Work out the finished part from the listing and answer in its coordinate system (mm). A direction names the side the tool comes from. Coordinates: 2 decimals unless noted, no trailing zeros. Order: outer loops, then holes, each group sorted by start corner. A loop starts at its lowest first (then second) coordinate and runs counter-clockwise, first axis right, second up. Notation, with made-up numbers: M 9.5,52 L 59.5,52 A32 ccw 59.5,83 Z; hole C 5,39 d7. An arc over 180 degrees is marked long. Write item = value, one per line. Start each with the question number.
Q1. Find section C-C on y = 1.2. Give the vertices of the cut face in (x, z).
Q2. Find section B-B on x = 3.75. Give the vertices of the cut face in (y, z), and give its area (4 significant figures).
Q3. A tool of negligible diameter and unlimited length cuts with its end or side. For faces 4 (the flat face through (7.5, 1, -51)), 5 (the cylindrical face through (3.8, 1.2, -97.5)), from which of +Z, -Z, +X, -X, +Y, -Y can it reach the whole face along a straight path? Write none if from no direction.
Q4. Determine the mould class of faces 1 (the cylindrical face through (3.67, 1.23, -103.75)), 2 (the flat face through (1.25, 1, -51)), 3 (the flat face through (0, 1, -49)) for opening direction Z: released by +Z, released by -Z, zero draft, split by the parting line, or undercut.
Q5. Straight lines are drawn through the part: line 1 along Z through (x, y) = (3.75, 0.7); line 2 along X through (y, z) = (1.95, -80); line 3 along Z through (x, y) = (3.25, 1.7). For each, find the intervals that lie inside material, in ascending order.
Q6. Find section A-A on z = -41.5. Give the vertices of the cut face in (x, y), and give its area (3 significant figures).
Q7. This flat-tipped pin is pushed along its axis until it touches: P1, Ø4, axis at x = 1.5, z = -40, coming from the -Y side. Where does it stop, or does it pass through?
```python
from build123d import *

# Parameters (mm, degrees)
SKETCH1_R           = 1.25
BOSS_EXTRUDE1_DEPTH = 2.5


with BuildPart() as part:
    # Sketch1 → Boss-Extrude1 (new body)
    with BuildSketch(Plane(origin=(0, 0, 0), x_dir=(1, 0, 0), z_dir=(0, 1, 0))):
        with BuildLine():
            Line((0, 0), (0, 100))
            ThreePointArc((0, 100), (3.75, 103.75), (7.5, 100))
            Line((7.5, 100), (7.5, 0))
            ThreePointArc((7.5, 0), (3.75, -3.75), (0, 0))
        make_face()
        with Locations((3.75, 0)):
            Circle(SKETCH1_R, mode=Mode.SUBTRACT)
        with Locations((3.75, 100)):
            Circle(SKETCH1_R, mode=Mode.SUBTRACT)
        with BuildLine():
            Line((1.25, 95), (1.25, 5))
            ThreePointArc((1.25, 5), (3.75, 2.5), (6.25, 5))
            Line((6.25, 5), (6.25, 95))
            ThreePointArc((6.25, 95), (3.75, 97.5), (1.25, 95))
        make_face(mode=Mode.SUBTRACT)
    extrude(amount=BOSS_EXTRUDE1_DEPTH)


solid = part.part
```
Findings below:
q1.outline = M 0,-100 A3.75 ccw 7.5,-100 L 7.5,0 A3.75 ccw 0,0 Z; hole M 1.25,-95 A2.5 ccw 6.25,-95 L 6.25,-5 A2.5 ccw 1.25,-5 Z; hole C 3.75,-100 d2.5; hole C 3.75,0 d2.5
q2.outline = M 0,-103.75 L 2.5,-103.75 L 2.5,-101.25 L 0,-101.25 Z; M 0,-98.75 L 2.5,-98.75 L 2.5,-97.5 L 0,-97.5 Z; M 0,-2.5 L 2.5,-2.5 L 2.5,-1.25 L 0,-1.25 Z; M 0,1.25 L 2.5,1.25 L 2.5,3.75 L 0,3.75 Z
q2.area = 18.75 mm^2
q3.face_4 = +Z, -Z, +X, +Y, -Y
q3.face_5 = +Y, -Y
q4.face_1 = released by -Z
q4.face_2 = undercut
q4.face_3 = zero draft
q5.line_1 = -103.75 to -101.25, -98.75 to -97.5, -2.5 to -1.25, 1.25 to 3.75
q5.line_2 = 0 to 1.25, 6.25 to 7.5
q5.line_3 = -103.72 to -101.15, -98.85 to -97.45, -2.55 to -1.15, 1.15 to 3.72
q6.outline = M 0,0 L 1.25,0 L 1.25,2.5 L 0,2.5 Z; M 6.25,0 L 7.5,0 L 7.5,2.5 L 6.25,2.5 Z
q6.area = 6.25 mm^2
q7.P1 = 0
